For this review, take the finished solid that the model builds, in its own axes (mm). Give positions to 0.01 mm unless a question says otherwise; leave off trailing zeros. Write each loop counter-clockwise with the first axis right and the second up, starting at its lowest first coordinate (ties: lowest second). Pieces come first, ordered by that corner, then holes. Notation, with made-up numbers: M 0,45 L 38,45 A28 cw 38,80 Z; hole C 35,52.5 d7. An arc over 180 degrees is marked long. One line per item, written item: value. Start each with the question number.
Item 1: Consider section D-D, the plane y = 26. Write out the cut boundary in (x, z) (1 decimal), and give its area (3 significant figures).
Item 2: Consider section C-C, the plane y = 12. Write out the cut boundary in (x, z) (1 decimal), and give its area (3 significant figures).
Item 3: Mouldability with a two-part tool opening along X and no side actions: class faces 1 (the face through (-7.31, 14.17, 5.6)), 2 (the face through (5, 0, 8)), 3 (the face through (1.323, 12.522, -10.074)) as released by +X, released by -X, zero draft, split by the parting line, or undercut.
Item 4: To check wall thickness, follow probe 1 along Z at (x, y) = (0, 20.75); probe 2 along X at (y, z) = (20.25, 6); probe 3 along Z at (x, y) = (-6.5, 19). State the ranges of each line that lie inside material, in increasing order.
Item 5: Clearance check with flat-ended pins moving along their axes: pin 1 Ø6 at (x, z) = (1, -4.5) entering from -Y; pin 2 Ø2 at (x, y) = (5, 12.5) entering from -Z; pin 3 Ø3 at (y, z) = (5, 5.5) entering from -X; pin 4 Ø1.5 at (y, z) = (14.5, 8) entering from +X. State where each tip first meets the part, or that it passes through.
Autodesk Inventor part; units mm, degrees
ref_plane "YZ Plane" through (0, 0, 0) normal (1, 0, 0) x (0, 1, 0)
ref_plane "XZ Plane" through (0, 0, 0) normal (0, 1, 0) x (-1, 0, 0)
ref_plane "XY Plane" through (0, 0, 0) normal (0, 0, 1) x (1, 0, 0)
sketch "Sketch1" plane through (0, 0, 0) normal (0, 1, 0) x (-1, 0, 0)
  circle A0 centre (0, 0) radius 10.16
  dimension "d0" = 20.32
extrude "Extrusion1" add sketch "Sketch1" along normal blind 25.4
sketch "Sketch2" plane through (0, 25.4, 0) normal (0, 1, 0) x (1, 0, 0)
  circle A0 centre (0, 0) radius 11.43
  dimension "d3" = 22.86
extrude "Extrusion2" add sketch "Sketch2" along normal blind 2.54
fillet "Fillet1" radius 1.27 2 edges at (-11.43, 25.4, 0) (-11.43, 27.94, 0)
sketch "Sketch3" plane through (0, 27.94, 0) normal (0, 1, 0) x (1, 0, 0)
  circle A0 centre (0, 0) radius 9.2075
  dimension "d7" = 18.415
extrude "Extrusion3" cut sketch "Sketch3" against normal blind 31.75
properties part number "Stack of train [Copy]"
Model answer:
1. outline: C 0,0 d22.5; hole C 0,0 d18.4
1. area: 130 mm2
2. outline: C 0,0 d20.3; hole C 0,0 d18.4
2. area: 58.0 mm2
3. face 1: undercut
3. face 2: zero draft
3. face 3: split by the parting line
4. probe 1: z = -10.16 to -9.21, 9.21 to 10.16
4. probe 2: x = -8.2 to -6.98, 6.98 to 8.2
4. probe 3: z = -7.81 to -6.52, 6.52 to 7.81
5. pin 1: passes through
5. pin 2: stops at z = -9.34
5. pin 3: stops at x = -9.34
5. pin 4: stops at x = 7.12
